Work out the finished part from the listing and answer in its coordinate system (mm). Face numbers are marked on the shaded views. A direction names the side the tool comes from. Give positions to 0.01 mm unless a question says otherwise; leave off trailing zeros. Write each loop counter-clockwise with the first axis right and the second up, starting at its lowest first coordinate (ties: lowest second). Pieces come first, ordered by that corner, then holes. Notation, with made-up numbers: (50.25, 53.5) - (103.25, 53.5) arc R26 cw to (103.25, 78.5) - close; hole circle Ø7 at (72, 26.25). An arc over 180 degrees is marked (long way). Write each question's results on one line, items separated by ' | '. Start each with the question number.
Autodesk Inventor part; units mm, degrees
ref_plane "YZ Plane" through (0, 0, 0) normal (1, 0, 0) x (0, 1, 0)
ref_plane "XZ Plane" through (0, 0, 0) normal (0, 1, 0) x (-1, 0, 0)
ref_plane "XY Plane" through (0, 0, 0) normal (0, 0, 1) x (1, 0, 0)
sketch "Sketch1" plane through (0, 0, 0) normal (0, 1, 0) x (-1, 0, 0)
  circle A0 centre (0, 0) radius 25
  dimension "d0" = 50
extrude "Extrusion1" add sketch "Sketch1" along normal blind 2
sketch "Sketch3" plane through (0, 2, 0) normal (0, 1, 0) x (1, 0, 0)
  circle A0 centre (0, 0) radius 27
  circle A1 centre (0, 0) radius 25
  dimension "d3" = 2
extrude "Extrusion2" add sketch "Sketch3" along normal blind 6.5 contours A0 | A1
sketch "Sketch4" plane through (0, 8.5, 0) normal (0, 1, 0) x (1, 0, 0)
  circle A0 centre (0, 0) radius 1.5
  circle A1 centre (-15, 15) radius 1
  dimension "d6" = 3
  dimension "d8" = 15
  dimension "d9" = 15
  dimension "d10" = 2
extrude "Extrusion3" cut sketch "Sketch4" against normal through all
sketch "Sketch5" plane through (0, 8.5, 0) normal (0, 1, 0) x (1, 0, 0)
  circle A0 centre (-15, 15) radius 3
  circle A1 centre (-15, 15) radius 1
  point P0 (0, 0)
  dimension "d14" = 2
extrude "Extrusion4" add sketch "Sketch5" along normal blind 10
thread "Thread1"
sketch "Sketch10" plane through (0, 0, 0) normal (0, -1, 0) x (1, 0, 0)
  circle A0 centre (9.5, 9.5) radius 11.5
  point P0 (0, 0)
  dimension "d31" = 23
  dimension "d32" = 9.5
  dimension "d33" = 9.5
extrude "Extrusion8" add sketch "Sketch10" along normal blind 20
sketch "Sketch11" plane through (9.5, -20, 9.5) normal (0, -1, 0) x (1, 0, 0)
  circle A0 centre (0, 0) radius 10.6
  circle A1 centre (0, 0) radius 11.5
  point P0 (-9.5, -9.5)
  dimension "d36" = 21.2
extrude "Extrusion9" cut sketch "Sketch11" against normal blind 2.5 contours A0
sketch "Sketch12" plane through (9.5, -17.5, 9.5) normal (0, -1, 0) x (1, 0, 0)
  circle A0 centre (0, 0) radius 7.4
  circle A1 centre (0, 0) radius 10.6
  point P0 (-9.5, -9.5)
  dimension "d39" = 14.8
extrude "Extrusion10" cut sketch "Sketch12" against normal through all contours A0
thread "Thread2"
properties part number "TopReactor"
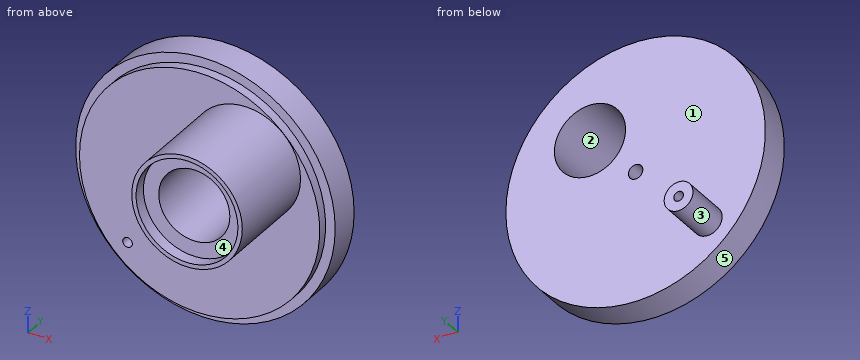
Q1. A cutting plane is placed at D-D, the plane x = -9. Write down the section's boundary in (y, z), and give its area (3 significant figures).
Q2. The mould has two halves that part along Z. Classify the marked faces 1, 2 and 3: pulls with the +Z half, pulls with the -Z half, needs draft (parallel to the pull), parting line crosses it, or undercut.
Q3. A cutting plane is placed at A-A, the plane z = 8.5. Write down the section's boundary in (x, y), and give its area (3 significant figures).
Q4. A tool of negligible diameter and unlimited length cuts with its end or side. For the marked faces 4 and 5, from which of +Z, -Z, +X, -X, +Y, -Y can it reach the whole face along a straight path? Write none if from no direction.
Q5. A cutting plane is placed at C-C, the plane y = 10. Write down the section's boundary in (x, z).
Q6. Consider L1, parallel to X at y = -7, z = 9; L2, parallel to Z at x = -15, y = 11.75; L3, parallel to Z at x = 9.5, y = -19.1. Determine where each line is inside the solid, lowest interval first.
Q7. Given pin 1 (4 mm diameter, centred on x = -5.5, z = 19.5, fed in from -Y); pin 2 (2 mm diameter, centred on x = 4, y = -6, fed in from +Z); pin 3 (2.5 mm diameter, centred on x = 0, z = 0, fed in from -Y); pin 4 (16 mm diameter, centred on x = 1.5, z = -9.5, fed in from +Y), each flat-ended and moving along its own axis, determine where each tip first touches the part or whether it passes through.
Q8. A cutting plane is placed at B-B, the plane x = 0. Write down the section's boundary in (y, z).
Result:
1) outline: (0, -23.32) - (2, -23.32) - (2, -25.46) - (8.5, -25.46) - (8.5, 25.46) - (2, 25.46) - (2, 23.32) - (0, 23.32) - close | area: 424 mm2
2) face 1: needs draft | face 2: undercut | face 3: parting line crosses it
3) outline: (-25.63, 2) - (-23.51, 2) - (-23.51, 0) - (-1.96, 0) - (-1.96, -20) - (-1.05, -20) - (-1.05, -17.5) - (2.17, -17.5) - (2.17, 8.5) - (-25.63, 8.5) - close; (16.83, -17.5) - (20.05, -17.5) - (20.05, -20) - (20.96, -20) - (20.96, 0) - (23.51, 0) - (23.51, 2) - (25.63, 2) - (25.63, 8.5) - (16.83, 8.5) - close | area: 451 mm2
4) face 4: -Y | face 5: +Y, -Y
5) outline: circle Ø6 at (-15, -15); hole circle Ø2 at (-15, -15)
6) L1: x = -1.99 to 2.12, 16.88 to 20.99 | L2: z = -18 to -16, -14 to -12 | L3: z = -2 to -1.1, 20.1 to 21
7) pin 1: stops at y = 0 | pin 2: stops at z = 20.08 | pin 3: passes through | pin 4: stops at y = 8.5
8) outline: (-20, 3.02) - (0, 3.02) - (0, 1.5) - (8.5, 1.5) - (8.5, 27) - (2, 27) - (2, 25) - (0, 25) - (0, 15.98) - (-20, 15.98) - (-20, 14.2) - (-17.5, 14.2) - (-17.5, 4.8) - (-20, 4.8) - close; (0, -25) - (2, -25) - (2, -27) - (8.5, -27) - (8.5, -1.5) - (0, -1.5) - close
